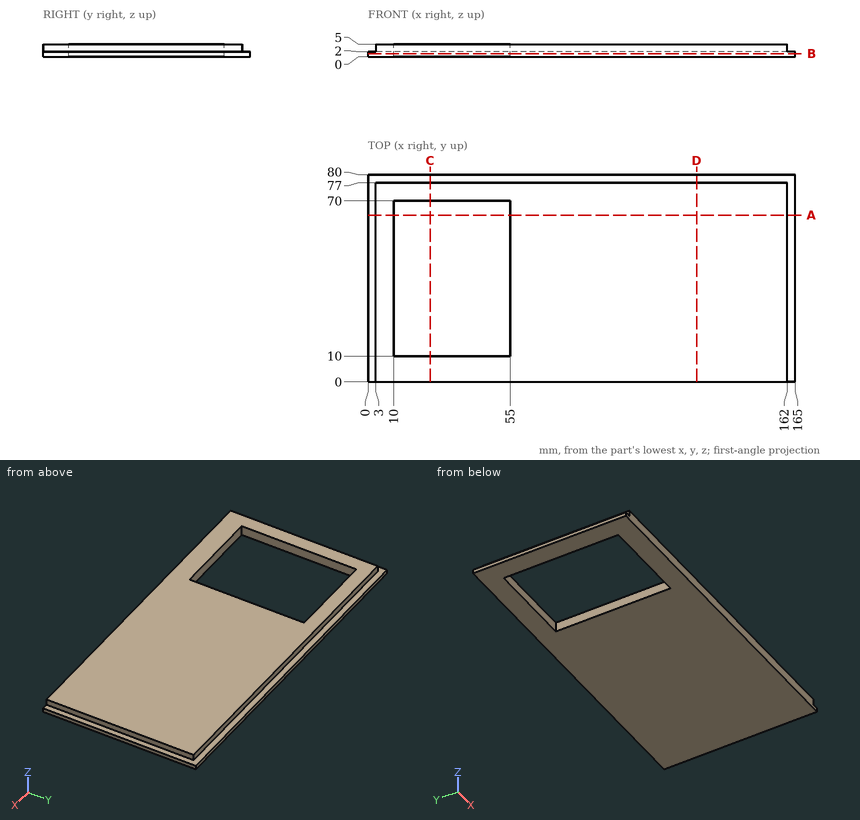
Could you check a few things on this drawing? It's one solid part, dimensions in mm from its lowest x, y, z. Round coordinates to 2 decimals unless told otherwise and drop trailing zeros. Loops run counter-clockwise (first coordinate to the right, second up) from the corner with the lowest first, then second, coordinate; pieces in that order, holes last.
Q1. Please list where these lines run through material, in increasing order: L1, parallel to X at y = 67, z = 2.75; L2, parallel to X at y = 50, z = 1.4; L3, parallel to Y at x = 13.5, z = 3.3.
Q2. For P1, Ø2.5, axis at y = 45.5, z = 3.5, coming from the -X side; P2, Ø1, axis at y = 69, z = 4.5, coming from the +X side, each with a flat end and sliding along its axis, tell me the tip position at first contact or that it passes through.
Q3. I want a section at C-C (x = 24). Write out the boundary of the cut face in (y, z), and give its area (3 significant figures).
Q4. I want a section at D-D (x = 127). Write out the boundary of the cut face in (y, z).
Q5. I want a section at B-B (z = 1.25). Write out the boundary of the cut face in (x, y), and give its area (3 significant figures).
Q6. I want a section at A-A (y = 64.5). Write out the boundary of the cut face in (x, z), and give its area (3 significant figures).
Answer below:
1. L1: x = 3 to 10, 55 to 162
1. L2: x = 0 to 10, 55 to 165
1. L3: y = 0 to 10, 70 to 77
2. P1: stops at x = 3
2. P2: stops at x = 162
3. outline: (0, 0) - (10, 0) - (10, 5) - (0, 5) - close; (70, 0) - (80, 0) - (80, 2) - (77, 2) - (77, 5) - (70, 5) - close
3. area: 91.0 mm2
4. outline: (0, 0) - (80, 0) - (80, 2) - (77, 2) - (77, 5) - (0, 5) - close
5. outline: (0, 0) - (165, 0) - (165, 80) - (0, 80) - close; hole (10, 10) - (55, 10) - (55, 70) - (10, 70) - close
5. area: 10,500 mm2
6. outline: (0, 0) - (10, 0) - (10, 5) - (3, 5) - (3, 2) - (0, 2) - close; (55, 0) - (165, 0) - (165, 2) - (162, 2) - (162, 5) - (55, 5) - close
6. area: 582 mm2
